Geometry check sheet. Reference: drawing and pictorial views, mm from the part's lowest x, y, z. Give positions to 0.01 mm unless a question says otherwise; leave off trailing zeros. Write each loop counter-clockwise with the first axis right and the second up, starting at its lowest first coordinate (ties: lowest second). Pieces come first, ordered by that corner, then holes. Notation, with made-up numbers: M 43.5,68.5 L 54.5,68.5 A18 ccw 54.5,91.5 Z; hole C 76,18.5 d4. An arc over 180 degrees is marked long. One line per item, written item: value. Start each with the question number.
1. Cross-section at C-C on z = 39.2. Record the cut outline in (x, y), then the cut area to 3 significant figures.
2. Cross-section at A-A on x = 55.7. Record the cut outline in (y, z), then the cut area to 3 significant figures.
3. Cross-section at B-B on y = 3.25. Record the cut outline in (x, z).
4. Gauge pin test, flat ends, axial feed: pin 1 (0.8 mm diameter, centred on x = 55, y = 6.5, fed in from -Z); pin 2 (1.5 mm diameter, centred on x = 15, z = 14.5, fed in from +Y); pin 3 (0.8 mm diameter, centred on y = 6, z = 13.5, fed in from -X); pin 4 (1.5 mm diameter, centred on y = 3, z = 40, fed in from +X). Record the tip position at first contact, or that the pin passes through.
5. Scan lines: line 1 (Z direction, x = 55.7, y = 1.9); line 2 (Y direction, x = 7, z = 38.5); line 3 (Z direction, x = 3, y = 7.25). Record each from-to range of solid material in increasing order.
6. Cross-section at D-D on x = 41.7. Record the cut outline in (y, z) (1 decimal), then the cut area to 3 significant figures.
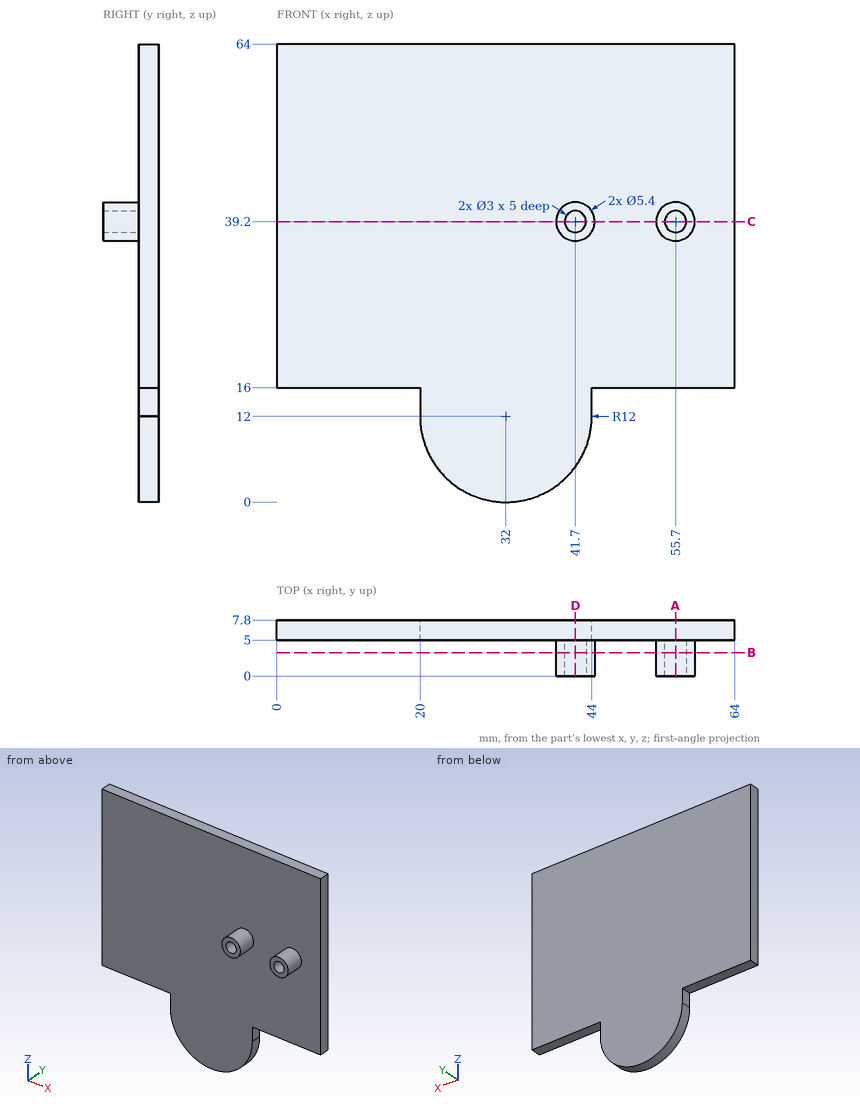
Report:
1. outline: M 0,5 L 39,5 L 39,0 L 40.2,0 L 40.2,5 L 43.2,5 L 43.2,0 L 44.4,0 L 44.4,5 L 53,5 L 53,0 L 54.2,0 L 54.2,5 L 57.2,5 L 57.2,0 L 58.4,0 L 58.4,5 L 64,5 L 64,7.8 L 0,7.8 Z
1. area: 203 mm^2
2. outline: M 0,36.5 L 5,36.5 L 5,16 L 7.8,16 L 7.8,64 L 5,64 L 5,41.9 L 0,41.9 L 0,40.7 L 5,40.7 L 5,37.7 L 0,37.7 Z
2. area: 146 mm^2
3. outline: C 41.7,39.2 d5.4; C 55.7,39.2 d5.4; hole C 41.7,39.2 d3; hole C 55.7,39.2 d3
4. pin 1: stops at z = 16
4. pin 2: passes through
4. pin 3: stops at x = 20
4. pin 4: stops at x = 58.4
5. line 1: z = 36.5 to 37.7, 40.7 to 41.9
5. line 2: y = 5 to 7.8
5. line 3: z = 16 to 64
6. outline: M 0,36.5 L 5,36.5 L 5,4.9 L 7.8,4.9 L 7.8,64 L 5,64 L 5,41.9 L 0,41.9 L 0,40.7 L 5,40.7 L 5,37.7 L 0,37.7 Z
6. area: 177 mm^2
